```python
from build123d import *

# Parameters (mm, degrees)
SKETCH1_R           = 1.6
BOSS_EXTRUDE1_DEPTH = 8
CHAMFER1_SIZE       = 1
SKETCH2_R           = 1.6
BOSS_EXTRUDE3_DEPTH = 8
FILLET1_R           = 2
CHAMFER5_SIZE       = 1


with BuildPart() as part:
    # Sketch1 → Boss-Extrude1 (new body)
    with BuildSketch(Plane.XY):
        with BuildLine():
            Line((-0.5, 3), (30.5, 3))
            ThreePointArc((30.5, 3), (32.267766953, 2.267766953), (33, 0.5))
            Line((33, 0.5), (33, -0.5))
            ThreePointArc((33, -0.5), (32.267766953, -2.267766953), (30.5, -3))
            Line((30.5, -3), (-0.5, -3))
            ThreePointArc((-0.5, -3), (-2.267766953, -2.267766953), (-3, -0.5))
            Line((-3, -0.5), (-3, 0.5))
            ThreePointArc((-3, 0.5), (-2.267766953, 2.267766953), (-0.5, 3))
        make_face()
        Circle(SKETCH1_R, mode=Mode.SUBTRACT)
        with Locations((7.5, 0)):
            Circle(SKETCH1_R, mode=Mode.SUBTRACT)
        with Locations((15, 0)):
            Circle(SKETCH1_R, mode=Mode.SUBTRACT)
        with Locations((22.5, 0)):
            Circle(SKETCH1_R, mode=Mode.SUBTRACT)
        with Locations((30, 0)):
            Circle(SKETCH1_R, mode=Mode.SUBTRACT)
    extrude(amount=BOSS_EXTRUDE1_DEPTH)

    # Chamfer1
    chamfer1_edges = [part.edges().sort_by_distance(p)[0] for p in [
        (-1.6, 0, 0),
        (-1.6, 0, 8),
        (5.9, 0, 0),
        (5.9, 0, 8),
        (13.4, 0, 0),
        (13.4, 0, 8),
        (20.9, 0, 0),
        (20.9, 0, 8),
        (28.4, 0, 0),
        (28.4, 0, 8),
    ]]
    chamfer(chamfer1_edges, length=CHAMFER1_SIZE)

    # Sketch2 → Boss-Extrude3 (add)
    with BuildSketch(Plane.XY.offset(8)):
        with BuildLine():
            ThreePointArc((-0.5, -3), (-2.267766953, -2.267766953), (-3, -0.5))
            Line((-3, -0.5), (-3, -23))
            ThreePointArc((-3, -23), (-2.267766953, -24.767766953), (-0.5, -25.5))
            Line((-0.5, -25.5), (0.5, -25.5))
            ThreePointArc((0.5, -25.5), (2.267766953, -24.767766953), (3, -23))
            Line((3, -23), (3, -3))
            Line((3, -3), (-0.5, -3))
        make_face()
        with Locations((0, -22.5)):
            Circle(SKETCH2_R, mode=Mode.SUBTRACT)
        with Locations((0, -15)):
            Circle(SKETCH2_R, mode=Mode.SUBTRACT)
        with Locations((0, -7.5)):
            Circle(SKETCH2_R, mode=Mode.SUBTRACT)
    extrude(amount=-BOSS_EXTRUDE3_DEPTH)

    # Fillet1
    fillet1_edges = [part.edges().sort_by_distance(p)[0] for p in [
        (3, -3, 4),
    ]]
    fillet(fillet1_edges, radius=FILLET1_R)

    # Chamfer5
    chamfer5_edges = [part.edges().sort_by_distance(p)[0] for p in [
        (-1.6, -7.5, 8),
        (-1.6, -15, 8),
        (-1.6, -22.5, 8),
        (-1.6, -22.5, 0),
        (-1.6, -15, 0),
        (-1.6, -7.5, 0),
    ]]
    chamfer(chamfer5_edges, length=CHAMFER5_SIZE)


solid = part.part
```
Geometry check sheet. Reference: the model listing, model coordinates, mm. Coordinates: 2 decimals unless noted, no trailing zeros. Order: outer loops, then holes, each group sorted by start corner. A loop starts at its lowest first (then second) coordinate and runs counter-clockwise, first axis right, second up. Notation, with made-up numbers: (60.25, 41) - (78.25, 41) arc R12 cw to (78.25, 62) - close; hole circle Ø9 at (-6.5, 45). An arc over 180 degrees is marked (long way). Answer in a Markdown table with one row per item. Add a question column.
1. Material ranges on L1, parallel to Y at x = 0, z = 4.1; L2, parallel to Y at x = 30, z = 3.3; L3, parallel to X at y = -18.5, z = 4.25, recorded low to high. Write a range as [from, to].
2. Gauge pin test, flat ends, axial feed: pin 1 Ø2 at (y, z) = (-18, 4) entering from +X; pin 2 Ø4 at (x, y) = (22.5, 0) entering from -Z. Record the tip position at first contact, or that the pin passes through.
3. Section check A-A (z = 6). Give the number of separate pieces and of enclosed holes in the cut face, plus the area to 3 significant figures.
4. Section check B-B (x = 7.5). Enter the section's corners in (y, z), plus the area to 3 significant figures.
5. Draft check along Y on faces 1 (the face through (18, -3, 4)), 2 (the face through (5.9, 0.07, 3.96)), 3 (the face through (6.9, -2.7, 8)). Enter one of: +Y half, -Y half, draft (parallel to the pull), parting line (faces both ways), or undercut.
Data:
| question | item | result |
|---|---|---|
| 1 | L1 | y = [-25.5, -24.1], [-20.9, -16.6], [-13.4, -9.1], [-5.9, -1.6], [1.6, 3] |
| 1 | L2 | y = [-3, -1.6], [1.6, 3] |
| 1 | L3 | x = [-3, 3] |
| 2 | pin 1 | stops at x = 3 |
| 2 | pin 2 | stops at z = 0.6 |
| 3 | separate pieces | 1 |
| 3 | enclosed holes | 8 |
| 3 | area | 281 mm² |
| 4 | outline | (-3, 0) - (-2.6, 0) - (-1.6, 1) - (-1.6, 7) - (-2.6, 8) - (-3, 8) - close; (1.6, 1) - (2.6, 0) - (3, 0) - (3, 8) - (2.6, 8) - (1.6, 7) - close |
| 4 | area | 20.4 mm² |
| 5 | face 1 | -Y half |
| 5 | face 2 | undercut |
| 5 | face 3 | draft |
